Verification items for this drawing (mm, ordinates from the low corner). A direction names the side the tool comes from. Coordinates: 2 decimals unless noted, no trailing zeros. Order: outer loops, then holes, each group sorted by start corner. A loop starts at its lowest first (then second) coordinate and runs counter-clockwise, first axis right, second up.
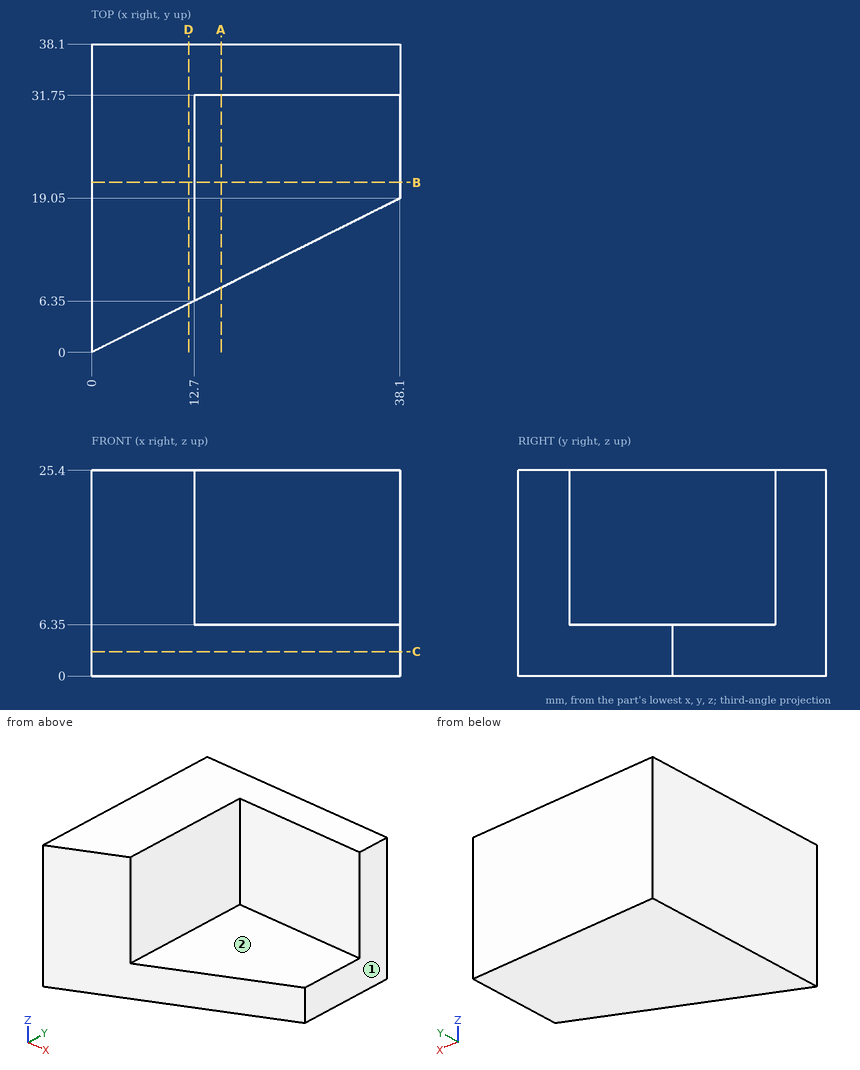
(1) Cross-section at C-C (z = 3). Enter the section's corners in (x, y).
Filled in:
outline: (0, 0) - (38.1, 19.05) - (38.1, 38.1) - (0, 38.1) - close
(2) Cross-section at B-B (y = 21). Enter the section's corners in (x, z), and give its area (3 significant figures).
Filled in:
outline: (0, 0) - (38.1, 0) - (38.1, 6.35) - (12.7, 6.35) - (12.7, 25.4) - (0, 25.4) - close
area: 484 mm2
(3) Thickness scan on probe 1 along X at (y, z) = (30, 7); probe 2 along Y at (x, z) = (33.5, 13.75); probe 3 along Z at (x, y) = (17, 27). Record the ranges inside material, lowest first.
Filled in:
probe 1: x = 0 to 12.7
probe 2: y = 31.75 to 38.1
probe 3: z = 0 to 6.35
(4) Cross-section at A-A (x = 16). Enter the section's corners in (y, z).
Filled in:
outline: (8, 0) - (38.1, 0) - (38.1, 25.4) - (31.75, 25.4) - (31.75, 6.35) - (8, 6.35) - close
(5) Go/stop test with flat-tipped pins: P1, Ø1, axis at x = 22, y = 9.5, coming from the +Z side; P2, Ø9.5, axis at x = 21.5, z = 12.5, coming from the -Y side; P3, Ø7.5, axis at x = 30, y = 17, coming from the +Z side; P4, Ø8, axis at y = 14.5, z = 15.5, coming from the +X side. Record where each tip stops, or that it passes through.
Filled in:
P1: passes through
P2: stops at y = 31.75
P3: stops at z = 6.35
P4: stops at x = 12.7
(6) Cross-section at D-D (x = 12). Enter the section's corners in (y, z).
Filled in:
outline: (6, 0) - (38.1, 0) - (38.1, 25.4) - (6, 25.4) - close
(7) Tool access check on the marked faces 1 and 2. Record the directions out of +Z, -Z, +X, -X, +Y, -Y that give a thin tool (end or side, any length) a straight path to the whole face; none if there is none.
Filled in:
face 1: +Z, -Z, +X, +Y, -Y
face 2: +Z, +X, -Y
